The listing builds one solid part. Answer for the finished solid, in the listing's coordinates (mm). A direction names the side the tool comes from. Give positions to 0.01 mm unless a question says otherwise; leave off trailing zeros. Loops run counter-clockwise (first coordinate to the right, second up) from the corner with the lowest first, then second, coordinate; pieces in that order, holes last. Notation, with made-up numbers: M -1.75,22.25 L 14.25,22.25 A22 cw 14.25,46.25 Z; hole C 47,13 d10. An arc over 180 degrees is marked long. One line per item, written item: value. Start each with the question number.
Q1. A flat-ended cylindrical pin translates along its axis: pin 1 (6.5 mm diameter, centred on x = -82.55, y = 82.55, fed in from +Z). Find the tip coordinate at first contact, or state that the pin passes through.
Q2. A cutting plane is placed at A-A, the plane y = -82.55. Determine the outline of the cut face in (x, z).
Q3. A cutting plane is placed at B-B, the plane x = 68. Determine the outline of the cut face in (y, z).
Q4. A cutting plane is placed at C-C, the plane z = 1. Determine the outline of the cut face in (x, y).
Q5. Consider L1, parallel to Y at x = 82.55, z = 4.5; L2, parallel to X at y = 26, z = 2.5. Determine where each line is inside the solid, lowest interval first.
Q6. For faces 1 (the flat face through (-1, 76.2, 3)), 2 (the flat face through (-88.9, -1, 3)), determine the directions among +Z, -Z, +X, -X, +Y, -Y from which every point of the face is accessible in a straight line to the end or side of a thin tool.
Q7. The mould has two halves that part along Y. Classify faces 3 (the cylindrical face through (-85.1, -82.4, 3.1)), 4 (the flat face through (88.9, -1, 3)), 5 (the flat face through (-1, 88.9, 3)): +Y half, -Y half, draft (parallel to the pull), parting line (faces both ways), or undercut.
from build123d import *

# Parameters (mm, degrees)
F0_W     = 177.8
F0_H     = 177.8
F0_R     = 2.5527
F0_W_2   = 152.4
F0_H_2   = 152.4
F1_DEPTH = 6.35


with BuildPart() as f1:
    # F0 (on Top) → F1 (new body)
    with BuildSketch(Plane.XY):
        Rectangle(F0_W, F0_H)
        with Locations((-82.55, -82.55)):
            Circle(F0_R, mode=Mode.SUBTRACT)
        with Locations((82.55, -82.55)):
            Circle(F0_R, mode=Mode.SUBTRACT)
        with Locations((-82.55, 82.55)):
            Circle(F0_R, mode=Mode.SUBTRACT)
        Rectangle(F0_W_2, F0_H_2, mode=Mode.SUBTRACT)
        with Locations((82.55, 82.55)):
            Circle(F0_R, mode=Mode.SUBTRACT)
    extrude(amount=F1_DEPTH)


solid = f1.part
Answer block:
1. pin 1: z = 6.35
2. outline: M -88.9,0 L -85.1,0 L -85.1,6.35 L -88.9,6.35 Z; M -80,0 L 80,0 L 80,6.35 L -80,6.35 Z; M 85.1,0 L 88.9,0 L 88.9,6.35 L 85.1,6.35 Z
3. outline: M -88.9,0 L -76.2,0 L -76.2,6.35 L -88.9,6.35 Z; M 76.2,0 L 88.9,0 L 88.9,6.35 L 76.2,6.35 Z
4. outline: M -88.9,-88.9 L 88.9,-88.9 L 88.9,88.9 L -88.9,88.9 Z; hole C -82.55,-82.55 d5.11; hole C -82.55,82.55 d5.11; hole M -76.2,-76.2 L 76.2,-76.2 L 76.2,76.2 L -76.2,76.2 Z; hole C 82.55,-82.55 d5.11; hole C 82.55,82.55 d5.11
5. L1: -88.9 to -85.1, -80 to 80, 85.1 to 88.9
5. L2: -88.9 to -76.2, 76.2 to 88.9
6. face 1: +Z, -Z
6. face 2: +Z, -Z, -X, +Y, -Y
7. face 3: undercut
7. face 4: draft
7. face 5: +Y half
